Verification items for the finished model (mm, model axes). A direction names the side the tool comes from. Give positions to 0.01 mm unless a question says otherwise; leave off trailing zeros. Order: outer loops, then holes, each group sorted by start corner. A loop starts at its lowest first (then second) coordinate and runs counter-clockwise, first axis right, second up. Notation, with made-up numbers: (6.5, 37) -> (13.5, 37) arc R22 ccw to (13.5, 59) -> close; hole circle Ø11 at (-2.5, 44.25). An arc over 180 degrees is marked (long way). Write each question's results on one line, items separated by ' | '. Start each with the question number.
1. Cross-section at A-A, the plane z = 77. Enter the section's corners in (x, y), then the cut area to 3 significant figures.
2. Depth check by flat-ended pin: pin 1 Ø3 at (x, z) = (4.5, 30.5) entering from +Y. Enter the tip coordinate at first touch or a pass-through.
3. Set-up check for faces 1 (the face through (14, 1.588, 104)), 2 (the face through (7, 1, -103.188)): record each of +Z, -Z, +X, -X, +Y, -Y from which the full face is reachable in a straight line by a thin tool's end or side.
4. Cross-section at B-B, the plane x = 17.25. Enter the section's corners in (y, z), then the cut area to 3 significant figures.
5. Material ranges on L1, parallel to Y at x = 21.25, z = 134, recorded low to high. Write a range as from..to.
from build123d import *

# Parameters (mm, degrees)
BOSS_EXTRUDE1_DEPTH = 304.8
FILLET1_R           = 0.254
CUT_EXTRUDE1_DEPTH  = 201.6125


with BuildPart() as part:
    # Sketch3 → Boss-Extrude1 (new, symmetric)
    with BuildSketch(Plane.XY):
        Polygon((1.5875, 25.4), (0, 25.4), (0, 0), (25.4, 0), (25.4, 1.5875), (1.5875, 1.5875), align=None)
    extrude(amount=BOSS_EXTRUDE1_DEPTH, both=True)

    # Fillet1
    fillet1_edges = [part.edges().sort_by_distance(p)[0] for p in [
        (1.5875, 1.5875, 0),
    ]]
    fillet(fillet1_edges, radius=FILLET1_R)

    # Sketch4 → Cut-Extrude1 (cut)
    with BuildSketch(Plane(origin=(0, 0, -304.8), x_dir=(-1, 0, 0), z_dir=(0, 0, -1))):
        with BuildLine():
            Line((-1.5875, 25.4), (-1.5875, 1.8415))
            ThreePointArc((-1.5875, 1.8415), (-1.661894878, 1.661894878), (-1.8415, 1.5875))
            Line((-1.8415, 1.5875), (-25.4, 1.5875))
            Line((-25.4, 1.5875), (-25.4, 0))
            Line((-25.4, 0), (0, 0))
            Line((0, 0), (0, 25.4))
            Line((0, 25.4), (-1.5875, 25.4))
        make_face()
    extrude(amount=-CUT_EXTRUDE1_DEPTH, mode=Mode.SUBTRACT)


solid = part.part
Results below:
1) outline: (0, 0) -> (25.4, 0) -> (25.4, 1.59) -> (1.84, 1.59) arc R0.25 cw to (1.59, 1.84) -> (1.59, 25.4) -> (0, 25.4) -> close | area: 78.1 mm²
2) pin 1: stops at y = 1.59
3) face 1: +Z, -Z, +X, +Y | face 2: -Z, +X, -X, +Y, -Y
4) outline: (0, -103.19) -> (1.59, -103.19) -> (1.59, 304.8) -> (0, 304.8) -> close | area: 648 mm²
5) L1: y = 0..1.59
